Check sheet for the drawn part. Datum: minimum x, y, z corner. Units: mm. Coordinates: 2 decimals unless noted, no trailing zeros. Write each loop counter-clockwise with the first axis right and the second up, starting at its lowest first coordinate (ties: lowest second). Pieces come first, ordered by that corner, then holes. Notation, with made-up numbers: (7, -8) - (14, -8) arc R19 ccw to (14, 14) - close; hole circle Ø6 at (79.25, 36.5). An arc over 180 degrees is marked (long way). Use one line per item in the form item = value. Start each with the question number.
1. Draft check along X on the marked faces 1, 2 and 3. Enter one of: +X half, -X half, draft (parallel to the pull), parting line (faces both ways), or undercut.
2. Cross-section at B-B on y = 50.8. Record the boundary of the cut face in (x, z), then the cut area to 3 significant figures.
3. Cross-section at C-C on z = 2.5. Record the boundary of the cut face in (x, y) (1 decimal), then the cut area to 3 significant figures.
4. Cross-section at D-D on x = 93. Record the boundary of the cut face in (y, z), then the cut area to 3 significant figures.
5. Go/stop test with flat-tipped pins: pin 1 Ø3 at (y, z) = (67.5, 5) entering from +X; pin 2 Ø1.5 at (y, z) = (17, 5) entering from -X; pin 3 Ø2 at (x, z) = (31, 3) entering from +Y. Record where each tip stops, or that it passes through.
6. Cross-section at A-A on x = 50.8. Record the boundary of the cut face in (y, z), then the cut area to 3 significant figures.
7. Scan lines: line 1 along X through (y, z) = (50.5, 4) (1 decimal); line 2 along X through (y, z) = (49.5, 4.5) (1 decimal); line 3 along Y through (x, z) = (46.5, 6) (1 decimal). Record each from-to range of solid material in increasing order.
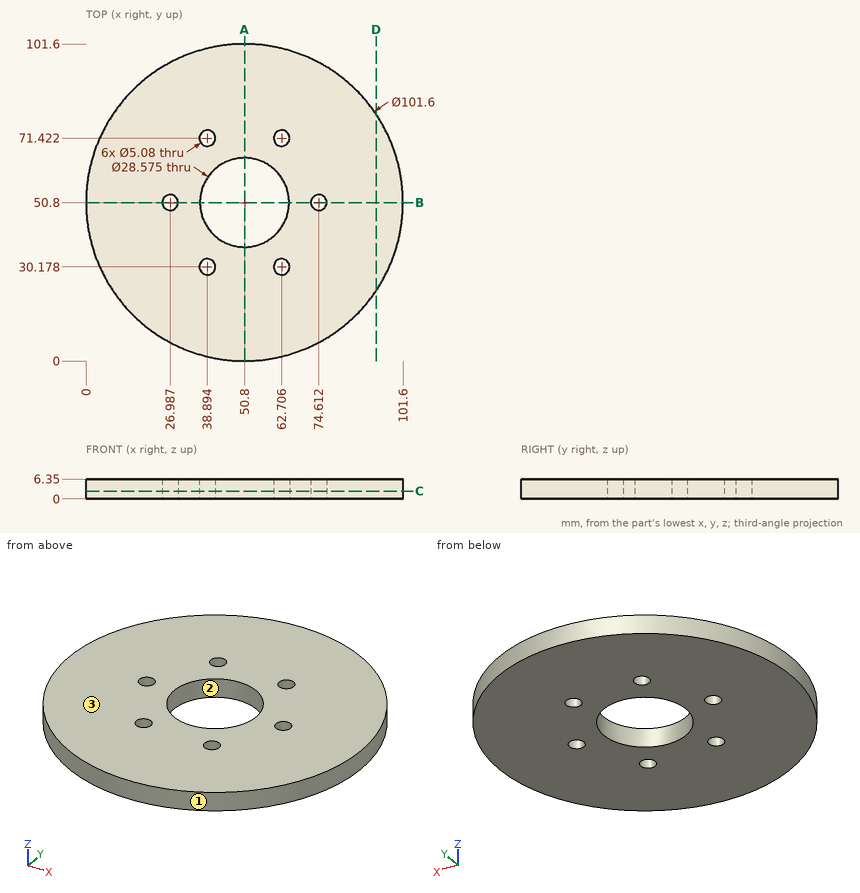
Final values:
q1.face_1 = parting line
q1.face_2 = undercut
q1.face_3 = draft
q2.outline = (0, 0) - (24.45, 0) - (24.45, 6.35) - (0, 6.35) - close; (29.53, 0) - (36.51, 0) - (36.51, 6.35) - (29.53, 6.35) - close; (65.09, 0) - (72.07, 0) - (72.07, 6.35) - (65.09, 6.35) - close; (77.15, 0) - (101.6, 0) - (101.6, 6.35) - (77.15, 6.35) - close
q2.area = 399 mm²
q3.outline = circle Ø101.6 at (50.8, 50.8); hole circle Ø5.1 at (27, 50.8); hole circle Ø5.1 at (38.9, 30.2); hole circle Ø5.1 at (38.9, 71.4); hole circle Ø28.6 at (50.8, 50.8); hole circle Ø5.1 at (62.7, 30.2); hole circle Ø5.1 at (62.7, 71.4); hole circle Ø5.1 at (74.6, 50.8)
q3.area = 7,340 mm²
q4.outline = (22.52, 0) - (79.08, 0) - (79.08, 6.35) - (22.52, 6.35) - close
q4.area = 359 mm²
q5.pin_1 = 99.27
q5.pin_2 = 12.22
q5.pin_3 = 97.99
q6.outline = (0, 0) - (36.51, 0) - (36.51, 6.35) - (0, 6.35) - close; (65.09, 0) - (101.6, 0) - (101.6, 6.35) - (65.09, 6.35) - close
q6.area = 464 mm²
q7.line_1 = 0 to 24.5, 29.5 to 36.5, 65.1 to 72.1, 77.1 to 101.6
q7.line_2 = 0 to 24.8, 29.2 to 36.6, 65 to 72.4, 76.8 to 101.6
q7.line_3 = 0.2 to 37.2, 64.4 to 101.4
